Read the model definition and answer for the solid it produces. Units are mm, in the model's axes. Face numbers are marked on the shaded views. A direction names the side the tool comes from. Give positions to 0.01 mm unless a question says otherwise; leave off trailing zeros. Order: outer loops, then holes, each group sorted by start corner. A loop starts at its lowest first (then second) coordinate and runs counter-clockwise, first axis right, second up. Notation, with made-up numbers: (33, -38.75) - (55, -38.75) arc R20 ccw to (55, -17.75) - close; hole circle Ø10 at (39.5, 71). An arc over 180 degrees is marked (long way). Return JSON: item names as keys, results as strings.
```python
from build123d import *

# Parameters (mm, degrees)
SKETCH1_R                    = 5.75
BOSS_EXTRUDE1_DEPTH          = 1
SKETCH2_R                    = 2.25
BOSS_EXTRUDE2_DEPTH          = 3
RIB2_REACH                   = 11.062
SKETCH3_WALL_W               = 24.654296494
SKETCH3_WALL_H               = 1
CHAMFER1_SIZE                = 0.3
CIRPATTERN1_COUNT            = 10
CHAMFER1_OF_CIRPATTERN1_SIZE = 0.3
SKETCH5_R                    = 2.5
BOSS_EXTRUDE4_DEPTH          = 0.5
SKETCH6_R                    = 1.5
CUT_EXTRUDE1_DEPTH           = 10.293815148
CUT_EXTRUDE2_DEPTH           = 9.667467912
CIRPATTERN2_COUNT            = 10


with BuildPart() as part:
    # Sketch1 → Boss-Extrude1 (new body)
    with BuildSketch(Plane(origin=(0, 0, 0), x_dir=(1, 0, 0), z_dir=(0, 1, 0))):
        with Locations(Location((0, 0, 0), (0, 0, 270))):
            Circle(SKETCH1_R)
    extrude(amount=BOSS_EXTRUDE1_DEPTH)

    # Sketch2 → Boss-Extrude2 (add)
    with BuildSketch(Plane(origin=(0, 1, 0), x_dir=(1, 0, 0), z_dir=(0, 1, 0))):
        with Locations(Location((0, 0, 0), (0, 0, 270))):
            Circle(SKETCH2_R)
    extrude(amount=BOSS_EXTRUDE2_DEPTH)

    # Sketch3 wall → Rib2 (add, up to next)
    with BuildSketch(Plane(origin=(-3.968577633, 2.475160602, 0), x_dir=(-0.758799561347, -0.651324209361, 0), z_dir=(0.651324209361, -0.758799561347, 0)), mode=Mode.PRIVATE) as rib2_sk1:
        Rectangle(SKETCH3_WALL_W, SKETCH3_WALL_H)
    rib2_tool1 = extrude(rib2_sk1.sketch, amount=RIB2_REACH, mode=Mode.PRIVATE) - part.part
    rib2 = rib2_tool1.solids().sort_by_distance((-3.968577633, 2.475160602, 0))[0]
    add(rib2)

    # Chamfer1
    chamfer1_edges = [part.edges().sort_by_distance(p)[0] for p in [
        (-3.940448181, 2.499305836, -0.5),
        (-3.940448181, 2.499305836, 0.5),
    ]]
    chamfer(chamfer1_edges, length=CHAMFER1_SIZE)

    # CirPattern1: Rib2 ×10 about axis
    cirpattern1_axis = Axis((0, 0, 0), (0, 1, 0))
    for i in range(1, CIRPATTERN1_COUNT):
        add(rib2.rotate(cirpattern1_axis, i * 360 / CIRPATTERN1_COUNT))

    # Chamfer1 of CirPattern1
    chamfer1_of_cirpattern1_edges = [part.edges().sort_by_distance(p)[0] for p in [
        (-3.48178217, 2.499305836, 1.911628831),
        (-2.893996918, 2.499305836, 2.720645826),
        (-1.693193712, 2.499305836, 3.593080423),
        (-0.742137195, 2.499305836, 3.902097417),
        (0.742137195, 2.499305836, 3.902097417),
        (1.693193712, 2.499305836, 3.593080423),
        (2.893996918, 2.499305836, 2.720645826),
        (3.48178217, 2.499305836, 1.911628831),
        (3.940448181, 2.499305836, 0.5),
        (3.940448181, 2.499305836, -0.5),
        (3.48178217, 2.499305836, -1.911628831),
        (2.893996918, 2.499305836, -2.720645826),
        (1.693193712, 2.499305836, -3.593080423),
        (0.742137195, 2.499305836, -3.902097417),
        (-0.742137195, 2.499305836, -3.902097417),
        (-1.693193712, 2.499305836, -3.593080423),
        (-2.893996918, 2.499305836, -2.720645826),
        (-3.48178217, 2.499305836, -1.911628831),
    ]]
    chamfer(chamfer1_of_cirpattern1_edges, length=CHAMFER1_OF_CIRPATTERN1_SIZE)

    # Sketch5 → Boss-Extrude4 (add)
    with BuildSketch(Plane.XZ):
        with Locations(Location((0, 0, 0), (0, 0, 270))):
            Circle(SKETCH5_R)
    extrude(amount=BOSS_EXTRUDE4_DEPTH)

    # Sketch6 → Cut-Extrude1 (cut, through all)
    with BuildSketch(Plane(origin=(0, 4, 0), x_dir=(1, 0, 0), z_dir=(0, 1, 0))):
        with Locations(Location((0, 0, 0), (0, 0, 270))):
            Circle(SKETCH6_R)
    extrude(amount=-CUT_EXTRUDE1_DEPTH, mode=Mode.SUBTRACT)

    # Sketch8 → Cut-Extrude2 (cut, through all)
    with BuildSketch(Plane(origin=(0, 1, 0), x_dir=(1, 0, 0), z_dir=(0, 1, 0))):
        with BuildLine():
            Line((-1.94763893, -5.347002675), (-1.567216323, -5.470609473))
            Line((-1.567216323, -5.470609473), (-1.139566108, -5.125257839))
            Line((-1.139566108, -5.125257839), (-0.828673564, -4.168428975))
            ThreePointArc((-0.828673564, -4.168428975), (0, -4.25), (0.828673564, -4.168428975))
            Line((0.828673564, -4.168428975), (1.139566108, -5.125257839))
            Line((1.139566108, -5.125257839), (1.567216323, -5.470609473))
            Line((1.567216323, -5.470609473), (1.649704909, -5.578945165))
            Line((1.649704909, -5.578945165), (0.683984218, -7.712906306))
            Line((0.683984218, -7.712906306), (-2.388981324, -6.322240681))
            Line((-2.388981324, -6.322240681), (-1.94763893, -5.347002675))
        make_face()
    cut_extrude2 = extrude(amount=-CUT_EXTRUDE2_DEPTH, mode=Mode.SUBTRACT)

    # CirPattern2: Cut-Extrude2 ×10 about axis
    cirpattern2_axis = Axis((0, 0, 0), (0, 1, 0))
    for i in range(1, CIRPATTERN2_COUNT):
        add(cut_extrude2.rotate(cirpattern2_axis, i * 360 / CIRPATTERN2_COUNT), mode=Mode.SUBTRACT)


solid = part.part
```
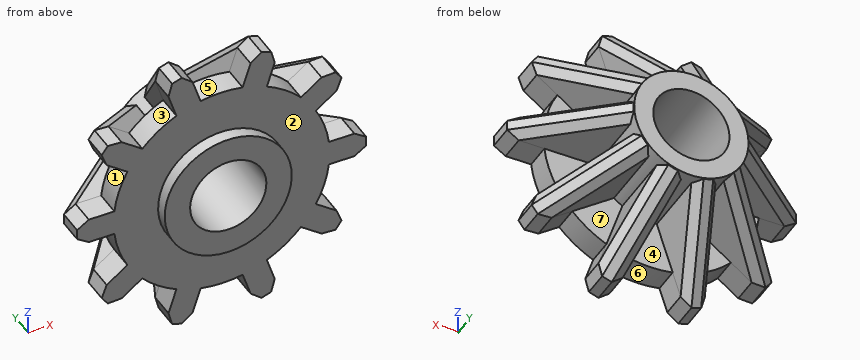
Q1. A cutting plane is placed at A-A (x = 0). Write down the section's boundary in (y, z).
Values:
{"outline": "(-0.5, -2.5) - (0, -2.5) - (0, -4.25) - (1, -4.25) - (1, -2.25) - (4, -2.25) - (4, -1.5) - (-0.5, -1.5) - close; (-0.5, 1.5) - (4, 1.5) - (4, 2.25) - (1, 2.25) - (1, 4.25) - (0, 4.25) - (0, 2.5) - (-0.5, 2.5) - close"}
Q2. Determine the mould class of the marked faces 4, 5, 6 and 7 for opening direction Z: released by +Z, released by -Z, zero draft, split by the parting line, or undercut.
Values:
{"face 4": "zero draft", "face 5": "released by +Z", "face 6": "released by -Z", "face 7": "undercut"}
Q3. Consider L1, parallel to X at y = 0.85, z = 3.25; L2, parallel to Z at x = -2.75, y = 2.7; L3, parallel to Z at x = 2.25, y = 2.6. Determine where each line is inside the solid, lowest interval first.
Values:
{"L1": "x = -4.67 to -3.62, -2.74 to 2.74, 3.62 to 4.67", "L2": "z = -2.33 to -1.38, -0.5 to 0.5, 1.38 to 2.33", "L3": "z = -2.25 to -1.02, -0.5 to 0.5, 1.02 to 2.25"}
Q4. For the marked faces 1, 2 and 3, determine the directions among +Z, -Z, +X, -X, +Y, -Y from which every point of the face is accessible in a straight line to the end or side of a thin tool.
Values:
{"face 1": "-X, +Y, -Y", "face 2": "-Y", "face 3": "+Y, -Y"}
Q5. Given pin 1 (0.8 mm diameter, centred on x = -3.5, z = 1, fed in from +Y); pin 2 (2 mm diameter, centred on x = -2, z = 3, fed in from +Y); pin 3 (0.5 mm diameter, centred on x = 5, y = 0.5, fed in from +Z), each flat-ended and moving along its own axis, determine where each tip first touches the part or whether it passes through.
Values:
{"pin 1": "stops at y = 1", "pin 2": "stops at y = 3.44", "pin 3": "stops at z = 0.5"}
Q6. A cutting plane is placed at B-B (z = 0). Write down the section's boundary in (x, y), and give its area (3 significant figures).
Values:
{"outline": "(-5.69, 0) - (-2.5, 0) - (-2.5, -0.5) - (-1.5, -0.5) - (-1.5, 4) - (-2.25, 4) - (-2.25, 3.95) - (-5.69, 1) - close; (1.5, -0.5) - (2.5, -0.5) - (2.5, 0) - (5.69, 0) - (5.69, 1) - (2.25, 3.95) - (2.25, 4) - (1.5, 4) - close", "area": "24.0 mm²"}
Q7. A cutting plane is placed at C-C (z = 4). Write down the section's boundary in (x, y), and give its area (3 significant figures).
Values:
{"outline": "(-1.83, 0) - (1.83, 0) - (1.83, 1.74) - (1.51, 2.22) - (1.09, 2.33) - (0.77, 2.02) - (0.77, 1) - (-0.77, 1) - (-0.77, 2.02) - (-1.09, 2.33) - (-1.51, 2.22) - (-1.83, 1.74) - close", "area": "6.08 mm²"}
